The listing builds one solid part. Answer for the finished solid, in the listing's coordinates (mm). Face numbers are marked on the shaded views. A direction names the side the tool comes from. Round coordinates to 2 decimals unless told otherwise and drop trailing zeros. Write each loop counter-clockwise with the first axis right and the second up, starting at its lowest first coordinate (ties: lowest second). Pieces come first, ordered by that corner, then holes.
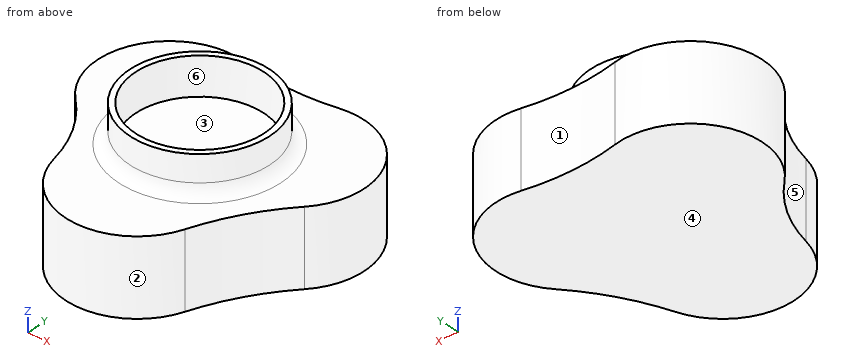
from build123d import *

# Parameters (mm, degrees)
PAD_DEPTH     = 20
SKETCH001_R   = 18.5
SKETCH001_R_2 = 17
PAD001_DEPTH  = 10
FILLET_R      = 3


with BuildPart() as part:
    # Sketch (on XY_Plane of Origin) → Pad (new body)
    with BuildSketch(Plane.XY):
        with BuildLine():
            ThreePointArc((30.707978, -3.063362), (32.870408, 19.066483), (12.550484, 28.094595))
            ThreePointArc((-12.550484, 28.094595), (0, 26.791295), (12.550484, 28.094595))
            ThreePointArc((-12.550484, 28.094595), (-33.317775, 18.253831), (-29.415109, -4.393248))
            ThreePointArc((-18.512219, -23.277607), (-22.553443, -13.021236), (-29.415109, -4.393248))
            ThreePointArc((-18.512219, -23.277607), (-0.927377, -37.977359), (18.006938, -25.062208))
            ThreePointArc((30.707978, -3.063362), (23.26018, -13.429271), (18.006938, -25.062208))
        make_face()
    extrude(amount=PAD_DEPTH)

    # Sketch001 (on Face8 of Pad) → Pad001 (join)
    with BuildSketch(Plane.XY.offset(20)):
        Circle(SKETCH001_R)
        Circle(SKETCH001_R_2, mode=Mode.SUBTRACT)
    extrude(amount=PAD001_DEPTH)

    # Fillet
    fillet_edges = [part.edges().sort_by_distance(p)[0] for p in [
        (-18.5, 0, 20),
    ]]
    fillet(fillet_edges, radius=FILLET_R)


solid = part.part
1. Section A-A on x = 0 is taken. Determine the outline of the cut face in (y, z), plus the area to 3 significant figures.
Geometry says:
outline: (-38, 0) - (26.79, 0) - (26.79, 20) - (21.5, 20) arc R3 cw to (18.5, 23) - (18.5, 30) - (17, 30) - (17, 20) - (-17, 20) - (-17, 30) - (-18.5, 30) - (-18.5, 23) arc R3 cw to (-21.5, 20) - (-38, 20) - close
area: 1,330 mm2
2. Section B-B on z = 27 is taken. Determine the outline of the cut face in (x, y), plus the area to 3 significant figures.
Geometry says:
outline: circle Ø37 at (0, 0); hole circle Ø34 at (0, 0)
area: 167 mm2
3. Section C-C on y = 0 is taken. Determine the outline of the cut face in (x, z), plus the area to 3 significant figures.
Geometry says:
outline: (-32.91, 0) - (32.91, 0) - (32.91, 20) - (21.5, 20) arc R3 cw to (18.5, 23) - (18.5, 30) - (17, 30) - (17, 20) - (-17, 20) - (-17, 30) - (-18.5, 30) - (-18.5, 23) arc R3 cw to (-21.5, 20) - (-32.91, 20) - close
area: 1,350 mm2
4. Given pin 1 (1.5 mm diameter, centred on x = -21, y = 5.5, fed in from +Z); pin 2 (5 mm diameter, centred on x = -13, z = 3.5, fed in from -Y); pin 3 (2 mm diameter, centred on y = 20.5, z = 7.5, fed in from +X), each flat-ended and moving along its own axis, determine where each tip first touches the part or whether it passes through.
Geometry says:
pin 1: stops at z = 20.05
pin 2: stops at y = -34.84
pin 3: stops at x = 32.61
5. A tool of negligible diameter and unlimited length cuts with its end or side. For the marked faces 5 and 6, from which of +Z, -Z, +X, -X, +Y, -Y can it reach the whole face along a straight path? Write none if from no direction.
Geometry says:
face 5: +Z, -Z, -X, -Y
face 6: +Z
6. Section D-D on z = 9 is taken. Determine the outline of the cut face in (x, y), plus the area to 3 significant figures.
Geometry says:
outline: (-29.42, -4.39) arc R37.31 cw to (-18.51, -23.28) arc R19 ccw to (18.01, -25.06) arc R64.29 cw to (30.71, -3.06) arc R19 ccw to (12.55, 28.09) arc R61.08 cw to (-12.55, 28.09) arc R19 ccw to start
area: 3,370 mm2
7. For a pull along X with two mould halves and no side action, classify the marked faces 1, 2, 3 and 4 as released by +X, released by -X, zero draft, split by the parting line, or undercut.
Geometry says:
face 1: undercut
face 2: split by the parting line
face 3: undercut
face 4: zero draft
8. Straight lines are drawn through the part: line 1 along Y through (x, z) = (0, 28.25); line 2 along Z through (x, y) = (-8.5, -13); line 3 along X through (y, z) = (6, 20.75). For each, find the intervals that lie inside material, in ascending order.
Geometry says:
line 1: y = -18.5 to -17, 17 to 18.5
line 2: z = 0 to 20
line 3: x = -18.57 to -15.91, 15.91 to 18.57
